from build123d import *

# Parameters (mm, degrees)
SKETCH5_W           = 76.2
SKETCH5_H           = 101.6
BOSS_EXTRUDE2_DEPTH = 25.4
BOSS_EXTRUDE3_DEPTH = 12.7
SKETCH8_R           = 38.1
BOSS_EXTRUDE4_DEPTH = 76.2
BOSS_EXTRUDE7_DEPTH = 76.2
SKETCH11_R          = 28.575
CUT_EXTRUDE3_DEPTH  = 135.861020279


with BuildPart() as part:
    # Sketch5 → Boss-Extrude2 (new body)
    with BuildSketch(Plane(origin=(0, 0, 0), x_dir=(1, 0, 0), z_dir=(0, 1, 0))):
        with Locations((0, 0.042847785)):
            Rectangle(SKETCH5_W, SKETCH5_H)
    extrude(amount=-BOSS_EXTRUDE2_DEPTH)

    # Sketch7 → Boss-Extrude3 (add, symmetric)
    with BuildSketch(Plane(origin=(0, 0, 0), x_dir=(0, 0, -1), z_dir=(1, 0, 0))):
        Polygon((-50.757152215, 0), (0.23059999, 56.627635701), (50.987752205, 56.627635701), (0, 0), align=None)
    extrude(amount=BOSS_EXTRUDE3_DEPTH, both=True)

    # Sketch8 → Boss-Extrude4 (add)
    with BuildSketch(Plane(origin=(0, 25.239549612, 28.031359668), x_dir=(1, 0, 0), z_dir=(0, 0.669130606, 0.743144825))):
        with Locations((0, 80.336835961)):
            Circle(SKETCH8_R)
    extrude(amount=-BOSS_EXTRUDE4_DEPTH)

    # Sketch14 → Boss-Extrude7 (add, through all)
    with BuildSketch(Plane(origin=(38.1, 0, 0), x_dir=(0, 0, -1), z_dir=(1, 0, 0))):
        Polygon((82.352111793, 33.953701348), (50.842847785, 0), (0, 0), (50.664048261, 56.26812605), (54.200329047, 60.078745736), align=None)
    extrude(amount=-BOSS_EXTRUDE7_DEPTH)

    # Sketch11 → Cut-Extrude3 (cut, through all)
    with BuildSketch(Plane(origin=(0, 25.239549612, 28.031359668), x_dir=(1, 0, 0), z_dir=(0, 0.669130606, 0.743144825))):
        with Locations((0, 80.336835961)):
            Circle(SKETCH11_R)
    extrude(amount=-CUT_EXTRUDE3_DEPTH, mode=Mode.SUBTRACT)


solid = part.part
The listing builds one solid part. Answer for the finished solid, in the listing's coordinates (mm). A direction names the side the tool comes from. Coordinates: 2 decimals unless noted, no trailing zeros. Order: outer loops, then holes, each group sorted by start corner. A loop starts at its lowest first (then second) coordinate and runs counter-clockwise, first axis right, second up.
Q1. Consider line 1 (Y direction, x = 16, z = 3.5); line 2 (Z direction, x = -3.5, y = 63.5); line 3 (Z direction, x = 18, y = 62). Determine where each line is inside the solid, lowest interval first.
Q2. Which of the six approach directions +Z, -Z, +X, -X, +Y, -Y give full straight-line access (tool end or side, diameter ignored) to faces 4 (the face through (-1, -13, -50.843)), 5 (the face through (-12.7, 22, 10)), 6 (the face through (25.58, 21.49, -19.35))?
Q3. A cutting plane is placed at B-B, the plane z = 31.5. Write down the section's boundary in (x, y).
Q4. A cutting plane is placed at D-D, the plane y = -3.5. Write down the section's boundary in (x, z), and give its area (3 significant figures).
Q5. A cutting plane is placed at C-C, the plane x = 32. Write down the section's boundary in (y, z).
Q6. A cutting plane is placed at A-A, the plane x = -10. Write down the section's boundary in (y, z), and give its area (3 significant figures).
Q7. Given P1, Ø7.5, axis at x = 19.5, z = 30, coming from the +Y side; P2, Ø6, axis at x = 28, z = -69.5, coming from the -Y side; P3, Ø1.5, axis at x = -4, z = -62.5, coming from the +Y side, each flat-ended and moving along its own axis, determine where each tip first touches the part or whether it passes through.
Q8. For a pull along Z with two mould halves and no side action, classify faces 1 (the face through (-0.838, 5.778, -56.719)), 2 (the face through (5.47, 106.05, -44.73)), 3 (the face through (-26, 0, 25)) as pulls with the +Z half, pulls with the -Z half, needs draft (parallel to the pull), parting line crosses it, or undercut.
Answers follow:
1. line 1: y = -25.4 to 0
1. line 2: z = -106.24 to -91.92, -7.15 to -6.42
1. line 3: z = -101.39 to -84.37, -18.04 to -5.07
2. face 4: -Z, +X, -X, -Y
2. face 5: +Z, -X
2. face 6: +Z, +X
3. outline: (-38.1, -25.4) - (38.1, -25.4) - (38.1, 0) - (12.7, 0) - (12.7, 21.39) - (-12.7, 21.39) - (-12.7, 0) - (-38.1, 0) - close
4. outline: (-38.1, -50.84) - (38.1, -50.84) - (38.1, 50.76) - (-38.1, 50.76) - close
4. area: 7,740 mm2
5. outline: (-25.4, -50.84) - (0, -50.84) - (18.79, -68.28) - (18.59, -68.52) - (49.32, -96.19) - (100.31, -39.56) - (69.57, -11.89) - (44.33, -39.92) - (0, 0) - (0, 50.76) - (-25.4, 50.76) - close
6. outline: (-25.4, -50.84) - (0, -50.84) - (7, -57.34) - (6.63, -57.75) - (14.06, -64.44) - (65.05, -7.81) - (57.62, -1.12) - (56.63, -2.23) - (56.63, -0.23) - (0, 50.76) - (-25.4, 50.76) - close; (53.85, -100.26) - (61.27, -106.95) - (112.26, -50.32) - (104.83, -43.64) - close
6. area: 7,390 mm2
7. P1: stops at y = 0
7. P2: stops at y = 16.35
7. P3: stops at y = 103.5
8. face 1: undercut
8. face 2: pulls with the +Z half
8. face 3: needs draft
